Source: CAD feature listing. Evaluate the final solid. Frame: model axes, mm. Face numbers are marked on the shaded views. A direction names the side the tool comes from. Give positions to 0.01 mm unless a question says otherwise; leave off trailing zeros. Write each loop counter-clockwise with the first axis right and the second up, starting at its lowest first coordinate (ties: lowest second). Pieces come first, ordered by that corner, then holes. Notation, with made-up numbers: M 62,62.5 L 73,62.5 A25 ccw 73,84.5 Z; hole C 27,-30 d11. An arc over 180 degrees is marked long. Return JSON: item names as keys, results as strings.
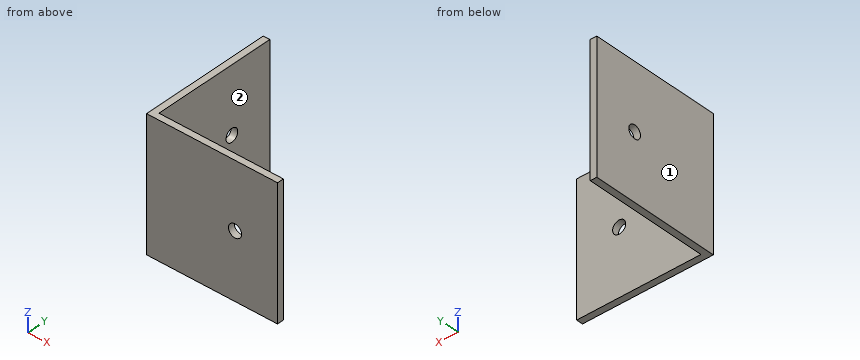
```python
from build123d import *

# Parameters (mm, degrees)
EXTRU_MINCE1_DEPTH      = 20
ESQUISSE2_R             = 1
ENL_V_MAT_EXTRU_1_DEPTH = 1
ESQUISSE3_R             = 1
ENL_V_MAT_EXTRU_2_DEPTH = 1


with BuildPart() as part:
    # Esquisse1 → Extru.-Mince1 (new body)
    with BuildSketch(Plane.XY):
        Polygon((0, 20), (0, 0), (20, 0), (20, 1), (1, 1), (1, 20), align=None)
    extrude(amount=EXTRU_MINCE1_DEPTH)

    # Esquisse2 → Enlèv. mat.-Extru.1 (cut)
    with BuildSketch(Plane(origin=(1, 0, 0), x_dir=(0, 0, -1), z_dir=(1, 0, 0))):
        with Locations((-10, 13.5)):
            Circle(ESQUISSE2_R)
    extrude(amount=-ENL_V_MAT_EXTRU_1_DEPTH, mode=Mode.SUBTRACT)

    # Esquisse3 → Enlèv. mat.-Extru.2 (cut)
    with BuildSketch(Plane(origin=(0, 1, 0), x_dir=(1, 0, 0), z_dir=(0, 1, 0))):
        with Locations(Location((13.5, -10, 0), (0, 0, 270))):
            Circle(ESQUISSE3_R)
    extrude(amount=-ENL_V_MAT_EXTRU_2_DEPTH, mode=Mode.SUBTRACT)


solid = part.part
```
1) Set-up query: the marked faces 1 and 2. Return all of +Z, -Z, +X, -X, +Y, -Y with unobstructed straight access to the full face (end or side cutting, diameter ignored); none if empty.
Numbers:
{"face 1": "+Z, -Z, -X, +Y, -Y", "face 2": "+Z, -Z, +X, +Y"}
2) Contact query for flat-ended pins moving along their axis: pin 1 Ø1.8 at (x, z) = (13.5, 10) entering from +Y; pin 2 Ø9.5 at (y, z) = (11, 12.5) entering from +X; pin 3 Ø9.5 at (x, z) = (8.5, 14.5) entering from +Y. Output: stop coordinate, or through.
Numbers:
{"pin 1": "passes through", "pin 2": "stops at x = 1", "pin 3": "stops at y = 1"}
3) Cut plane D-D, the plane z = 16.25. Return the cut outline in (x, y), then the cut area to 3 significant figures.
Numbers:
{"outline": "M 0,0 L 20,0 L 20,1 L 1,1 L 1,20 L 0,20 Z", "area": "39.0 mm²"}
4) Cut plane C-C, the plane z = 10. Return the cut outline in (x, y).
Numbers:
{"outline": "M 0,0 L 12.5,0 L 12.5,1 L 1,1 L 1,12.5 L 0,12.5 Z; M 0,14.5 L 1,14.5 L 1,20 L 0,20 Z; M 14.5,0 L 20,0 L 20,1 L 14.5,1 Z"}
5) Line query: line 1 (X direction, y = 0.8, z = 10); line 2 (X direction, y = 5.5, z = 11.25). Output: solid intervals per line, ascending. Write a range as [from, to].
Numbers:
{"line 1": "x = [0, 12.5], [14.5, 20]", "line 2": "x = [0, 1]"}
6) Cut plane A-A, the plane x = 13.5. Return the cut outline in (y, z), then the cut area to 3 significant figures.
Numbers:
{"outline": "M 0,0 L 1,0 L 1,9 L 0,9 Z; M 0,11 L 1,11 L 1,20 L 0,20 Z", "area": "18.0 mm²"}
